from build123d import *

# Parameters (mm, degrees)
EXTRUDE_1_DEPTH      = 3
EXTRUDE_1_DEPTH_BACK = 3
SKETCH_1_R           = 2
SKETCH_1_R_2         = 1
SKETCH_2_W           = 130
SKETCH_2_H           = 40
EXTRUDE_2_DEPTH      = 10
SKETCH_3_W           = 41
SKETCH_3_H           = 20
CUT_EXTRUDE_1_DEPTH  = 10
FILLET_1_R           = 10
HOLE_WIZARD_M3_1_D   = 3.4
FILLET_4_R           = 10


with BuildPart() as part:
    # 스케치1 → 보스-돌출1 (new, two sides: drawn at the far end of the back side and taken through both)
    with BuildSketch(Plane.XY.offset(-EXTRUDE_1_DEPTH_BACK)):
        with BuildLine():
            Line((0, 20), (45, 20))
            Line((45, 20), (45, -20))
            Line((45, -20), (0, -20))
            ThreePointArc((0, -20), (-20, 0), (0, 20))
        make_face()
        Circle(SKETCH_1_R, mode=Mode.SUBTRACT)
        with Locations((0, 16.16)):
            Circle(SKETCH_1_R_2, mode=Mode.SUBTRACT)
        with Locations((16.16, 0)):
            Circle(SKETCH_1_R_2, mode=Mode.SUBTRACT)
        with Locations((0, -16.16)):
            Circle(SKETCH_1_R_2, mode=Mode.SUBTRACT)
        with Locations((-16.16, 0)):
            Circle(SKETCH_1_R_2, mode=Mode.SUBTRACT)
    extrude(amount=EXTRUDE_1_DEPTH + EXTRUDE_1_DEPTH_BACK)

    # 스케치2 → 보스-돌출2 (add)
    with BuildSketch(Plane(origin=(45, 0, 0), x_dir=(0, 0, -1), z_dir=(1, 0, 0))):
        Rectangle(SKETCH_2_W, SKETCH_2_H)
    extrude(amount=EXTRUDE_2_DEPTH)

    # 스케치3 → 컷-돌출1 (cut)
    with BuildSketch(Plane(origin=(55, 0, 0), x_dir=(0, 0, -1), z_dir=(1, 0, 0))):
        with Locations((32.5, 10)):
            Rectangle(SKETCH_3_W, SKETCH_3_H)
        with Locations((-32.5, 10)):
            Rectangle(SKETCH_3_W, SKETCH_3_H)
    extrude(amount=-CUT_EXTRUDE_1_DEPTH, mode=Mode.SUBTRACT)

    # 필렛1
    fillet_1_edges = [part.edges().sort_by_distance(p)[0] for p in [
        (55, -20, 0),
    ]]
    fillet(fillet_1_edges, radius=FILLET_1_R)

    # M3 여유 구멍1 (through all)
    with Locations(Plane(origin=(55, 0, 0), x_dir=(0, 0, -1), z_dir=(1, 0, 0))):
        with Locations((-57.8, 14.5), (-57.8, 5.5), (-7.5, 14.5), (-7.5, 5.5), (7.2, 14.5), (7.2, 5.5), (57.5, 14.5), (57.5, 5.5)):
            Hole(HOLE_WIZARD_M3_1_D / 2)

    # 필렛4
    fillet_4_edges = [part.edges().sort_by_distance(p)[0] for p in [
        (50, 20, -65),
        (50, 20, 65),
    ]]
    fillet(fillet_4_edges, radius=FILLET_4_R)


solid = part.part
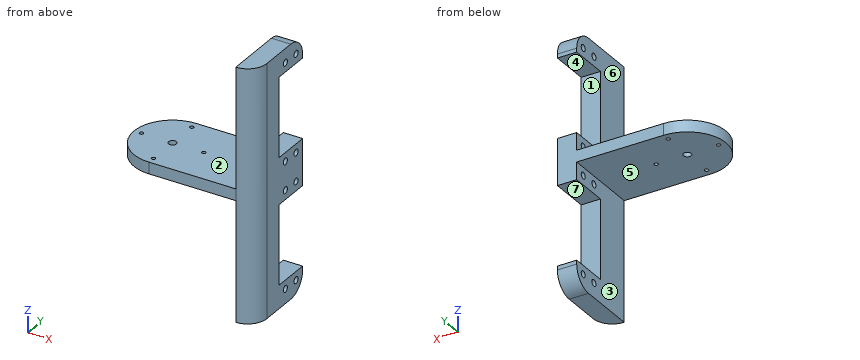
The listing builds one solid part. Answer for the finished solid, in the listing's coordinates (mm). Face numbers are marked on the shaded views. A direction names the side the tool comes from. Give positions to 0.01 mm unless a question says otherwise; leave off trailing zeros. Order: outer loops, then holes, each group sorted by start corner. A loop starts at its lowest first (then second) coordinate and runs counter-clockwise, first axis right, second up. Notation, with made-up numbers: (76, 30) - (80, 30) arc R18 cw to (80, 39) - close; hole circle Ø4 at (29.25, 48). An arc over 180 degrees is marked (long way). Answer as CSV lines item,"result".
Q1. A cutting plane is placed at B-B, the plane x = 27.5. Determine the outline of the cut face in (y, z).
Answer key:
outline,"(-20, -3) - (20, -3) - (20, 3) - (-20, 3) - close"
Q2. A cutting plane is placed at A-A, the plane z = -7.2. Determine the outline of the cut face in (x, y), and give its area (3 significant figures).
Answer key:
outline,"(45, -20) arc R10 ccw to (55, -10) - (55, 3.8) - (45, 3.8) - close; (45, 7.2) - (55, 7.2) - (55, 12.8) - (45, 12.8) - close; (45, 16.2) - (55, 16.2) - (55, 20) - (45, 20) - close"
area,"311 mm^2"
Q3. A cutting plane is placed at D-D, the plane z = 37. Determine the outline of the cut face in (x, y).
Answer key:
outline,"(45, -20) arc R10 ccw to (55, -10) - (55, 0) - (45, 0) - close"
Q4. A cutting plane is placed at C-C, the plane z = 57.8. Determine the outline of the cut face in (x, y).
Answer key:
outline,"(45, -20) arc R10 ccw to (55, -10) - (55, 3.8) - (45, 3.8) - close; (45, 7.2) - (55, 7.2) - (55, 12.8) - (45, 12.8) - close; (45, 16.2) - (55, 16.2) - (55, 19.6) - (45, 19.6) - close"
Q5. Which of the six approach directions +Z, -Z, +X, -X, +Y, -Y give full straight-line access (tool end or side, diameter ignored) to the marked faces 5, 6 and 7?
Answer key:
face 5,"-Z, -X, +Y, -Y"
face 6,"+Z, -X, +Y, -Y"
face 7,"+X, -X, +Y"
Q6. Each of these flat-tipped pins is pushed along its axis until it touches: pin 1 Ø20 at (x, y) = (13, 8) entering from +Z; pin 2 Ø12 at (y, z) = (0, 37.5) entering from -X; pin 3 Ø5 at (x, z) = (50.5, 37.5) entering from +Y; pin 4 Ø2 at (y, z) = (14.5, -57.5) entering from +X. Where does it stop, or does it pass through?
Answer key:
pin 1,"stops at z = 3"
pin 2,"stops at x = 45"
pin 3,"stops at y = 0"
pin 4,"passes through"
Q7. Straight lines are drawn through the part: L1, parallel to Y at x = 0, z = -0.85; L2, parallel to Z at x = 36, y = 14; L3, parallel to Y at x = 52, z = 57. For each, find the intervals that lie inside material, in ascending order.
Answer key:
L1,"y = -20 to -17.16, -15.16 to -2, 2 to 15.16, 17.16 to 20"
L2,"z = -3 to 3"
L3,"y = -17.14 to 4, 7 to 13, 16 to 19.8"
Q8. Determine the mould class of the marked faces 1, 2, 3 and 4 for opening direction Z: pulls with the +Z half, pulls with the -Z half, needs draft (parallel to the pull), parting line crosses it, or undercut.
Answer key:
face 1,"undercut"
face 2,"pulls with the +Z half"
face 3,"needs draft"
face 4,"undercut"
